The model under review builds one solid part; all positions refer to its coordinate system, in mm. Round coordinates to 2 decimals unless told otherwise and drop trailing zeros. Write each loop counter-clockwise with the first axis right and the second up, starting at its lowest first coordinate (ties: lowest second). Pieces come first, ordered by that corner, then holes. Notation, with made-up numbers: (-29, 42.5) -> (18, 42.5) arc R28 ccw to (18, 61.5) -> close; hole circle Ø9 at (15.25, 82.5). An arc over 180 degrees is marked (long way). Answer as a JSON object with one key per item and string values. Group by question number.
1) We need section B-B, the plane y = 13. Write out the cut boundary in (x, z), then the cut area to 3 significant figures.
2) Insertion check: pin 1 Ø5 at (x, y) = (-42, 21.5) entering from -Z; pin 2 Ø12 at (x, z) = (48.5, -57.5) entering from +Y; pin 3 Ø0.6 at (y, z) = (1, -74) entering from -X. Each pin has a flat end and moves straight along its axis. Give the tip position at first contact, or say it passes through.
3) To check wall thickness, follow probe 1 along X at (y, z) = (0.85, -72.5); probe 2 along Z at (x, y) = (19.5, 0.5); probe 3 along Y at (x, z) = (12, 59.5). State the ranges of each line that lie inside material, in increasing order. Write a range as [from, to].
4) We need section D-D, the plane x = -51.5. Write out the cut boundary in (y, z) (3 decimals).
5) We need section A-A, the plane x = -19.5. Write out the cut boundary in (y, z).
6) We need section C-C, the plane z = -35. Write out the cut boundary in (x, y), then the cut area to 3 significant figures.
from build123d import *

# Parameters (mm, degrees)
BOSS_EXTRUDE1_DEPTH = 2
CUT_EXTRUDE1_REACH  = 4
SKETCH2_R           = 2
BOSS_EXTRUDE2_DEPTH = 2
CUT_EXTRUDE2_REACH  = 4
SKETCH5_R           = 1.5
SKETCH6_R           = 2.5
BOSS_EXTRUDE3_DEPTH = 30


with BuildPart() as part:
    # Sketch1 → Boss-Extrude1 (new body)
    with BuildSketch(Plane(origin=(0, 0, 0), x_dir=(1, 0, 0), z_dir=(0, 1, 0))):
        Polygon((-75, -70), (-65, -80), (65, -80), (75, -70), (75, -30), (35, 80), (-35, 80), (-75, -30), align=None)
    extrude(amount=BOSS_EXTRUDE1_DEPTH)

    # Sketch2 → Cut-Extrude1 (cut, up to next)
    with BuildSketch(Plane.XZ, mode=Mode.PRIVATE) as cut_extrude1_sk1:
        with Locations((-19.5, -50.31270399)):
            Circle(SKETCH2_R)
    cut_extrude1_tool1 = extrude(cut_extrude1_sk1.sketch, amount=-CUT_EXTRUDE1_REACH, mode=Mode.PRIVATE) & part.part
    add(cut_extrude1_tool1.solids().sort_by_distance((-19.5, 0, -50.312704))[0], mode=Mode.SUBTRACT)
    # Sketch2 → Cut-Extrude1 (cut, up to next)
    with BuildSketch(Plane.XZ, mode=Mode.PRIVATE) as cut_extrude1_sk2:
        with Locations((19.5, -50.31270399)):
            Circle(SKETCH2_R)
    cut_extrude1_tool2 = extrude(cut_extrude1_sk2.sketch, amount=-CUT_EXTRUDE1_REACH, mode=Mode.PRIVATE) & part.part
    add(cut_extrude1_tool2.solids().sort_by_distance((19.5, 0, -50.312704))[0], mode=Mode.SUBTRACT)

    # Sketch3 → Boss-Extrude2 (add)
    with BuildSketch(Plane.XZ):
        Polygon((-35, -80), (-60, -80), (-60, -67.5), (60, -67.5), (60, -80), align=None)
    extrude(amount=-BOSS_EXTRUDE2_DEPTH)

    # Sketch5 → Cut-Extrude2 (cut, up to next)
    with BuildSketch(Plane(origin=(0, 2, 0), x_dir=(1, 0, 0), z_dir=(0, 1, 0)), mode=Mode.PRIVATE) as cut_extrude2_sk1:
        with Locations((57, 72.5)):
            Circle(SKETCH5_R)
    cut_extrude2_tool1 = extrude(cut_extrude2_sk1.sketch, amount=-CUT_EXTRUDE2_REACH, mode=Mode.PRIVATE) & part.part
    add(cut_extrude2_tool1.solids().sort_by_distance((57, 2, -72.5))[0], mode=Mode.SUBTRACT)
    # Sketch5 → Cut-Extrude2 (cut, up to next)
    with BuildSketch(Plane(origin=(0, 2, 0), x_dir=(1, 0, 0), z_dir=(0, 1, 0)), mode=Mode.PRIVATE) as cut_extrude2_sk2:
        with Locations((-57, 72.5)):
            Circle(SKETCH5_R)
    cut_extrude2_tool2 = extrude(cut_extrude2_sk2.sketch, amount=-CUT_EXTRUDE2_REACH, mode=Mode.PRIVATE) & part.part
    add(cut_extrude2_tool2.solids().sort_by_distance((-57, 2, -72.5))[0], mode=Mode.SUBTRACT)

    # Sketch6 → Boss-Extrude3 (add)
    with BuildSketch(Plane(origin=(0, 2, 0), x_dir=(1, 0, 0), z_dir=(0, 1, 0))):
        with Locations((-40, -20.935279196)):
            Circle(SKETCH6_R)
        with Locations((40, -20.935279196)):
            Circle(SKETCH6_R)
        with Locations((0, 35)):
            Circle(SKETCH6_R)
    extrude(amount=BOSS_EXTRUDE3_DEPTH)


solid = part.part
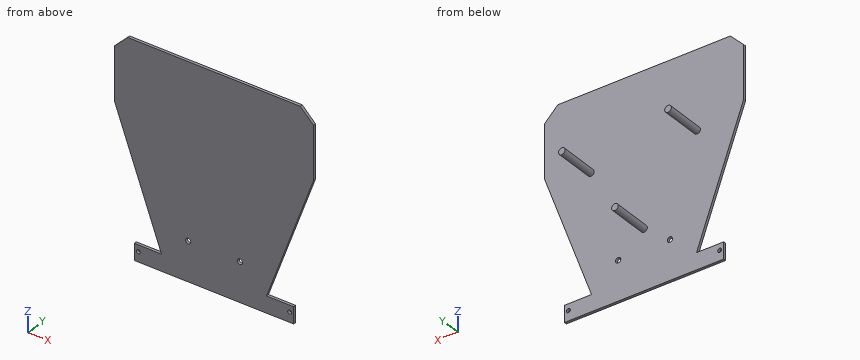
Here are the results:
{
 "1": {"outline": "circle Ø5 at (-40, 20.94); circle Ø5 at (0, -35); circle Ø5 at (40, 20.94)", "area": "58.9 mm^2"},
 "2": {"pin 1": "stops at z = 18.44", "pin 2": "stops at y = 2", "pin 3": "stops at x = -60"},
 "3": {"probe 1": "x = [-60, -58.5], [-55.5, 55.5], [58.5, 60]", "probe 2": "z = [-80, -52.31], [-48.31, 80]", "probe 3": "y = [0, 2]"},
 "4": {"outline": "(0, -80) -> (2, -80) -> (2, -67.5) -> (0, -67.5) -> close; (0, -34.625) -> (2, -34.625) -> (2, 80) -> (0, 80) -> close"},
 "5": {"outline": "(0, -80) -> (2, -80) -> (2, -52.31) -> (0, -52.31) -> close; (0, -48.31) -> (2, -48.31) -> (2, 80) -> (0, 80) -> close"},
 "6": {"outline": "(-51.36, 0) -> (51.36, 0) -> (51.36, 2) -> (2.5, 2) -> (2.5, 32) -> (-2.5, 32) -> (-2.5, 2) -> (-51.36, 2) -> close", "area": "355 mm^2"}
}
